Answer from the drawing. Dimensions are ordinates in mm from the lowest x, y and z of the part. Coordinates: 2 decimals unless noted, no trailing zeros. Order: outer loops, then holes, each group sorted by start corner. A loop starts at its lowest first (then second) coordinate and runs counter-clockwise, first axis right, second up. Notation, with made-up numbers: (76, -36) -> (103, -36) arc R16 cw to (103, -14) -> close; hole circle Ø5 at (18.25, 2). An arc over 180 degrees is marked (long way). Answer in a Markdown table with one row per item.
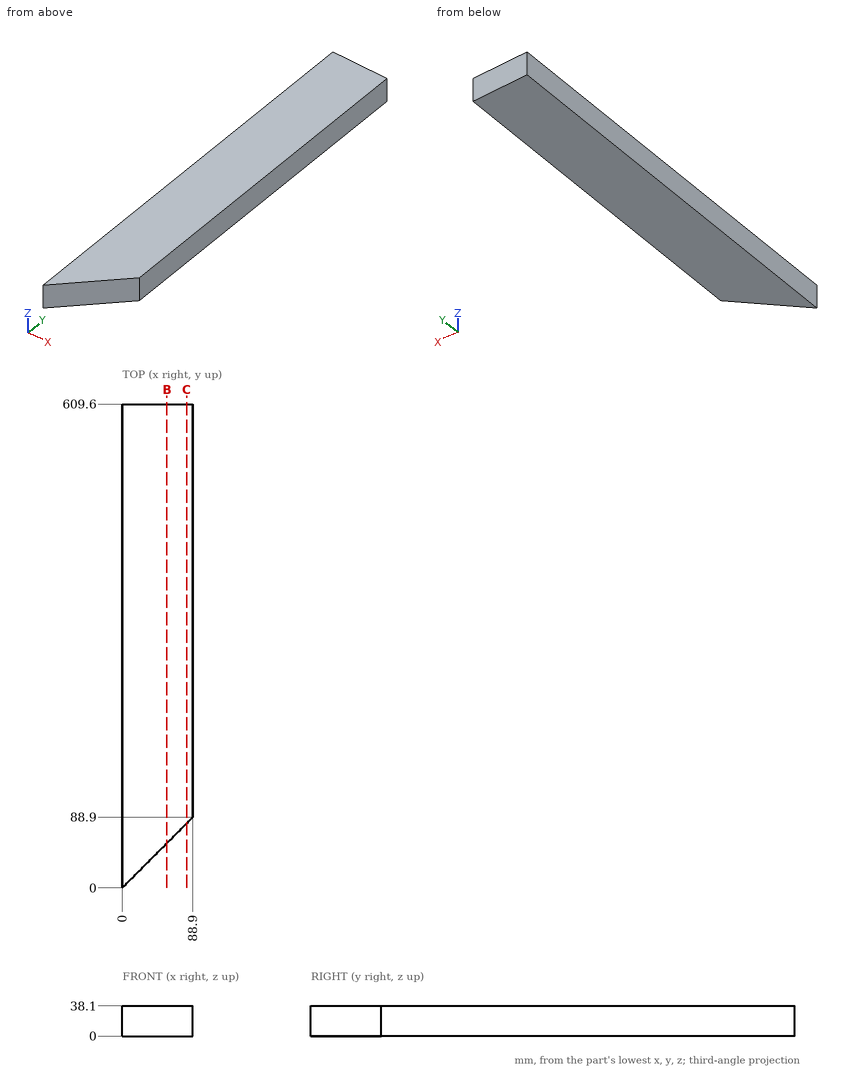
(1) Flat-ended cylindrical pins translate along their axes: pin 1 (8 mm diameter, centred on y = 547.5, z = 18, fed in from -X); pin 2 (3 mm diameter, centred on y = 70, z = 25.5, fed in from +X); pin 3 (4 mm diameter, centred on x = 28.5, z = 4.5, fed in from -Y). Find the tip coordinate at first contact, or state that the pin passes through.
Check values:
| item | result |
|---|---|
| pin 1 | x = 0 |
| pin 2 | x = 71.5 |
| pin 3 | y = 26.5 |
(2) Find the intervals of material crossed by line 1 along Y through (x, z) = (62.5, 18.5); line 2 along Y through (x, z) = (26.5, 8); line 3 along X through (y, z) = (51, 27), in increasing order. Write a range as from..to.
Check values:
| item | result |
|---|---|
| line 1 | 62.5..609.6 |
| line 2 | 26.5..609.6 |
| line 3 | 0..51 |
(3) A cutting plane is placed at B-B, the plane x = 56. Determine the outline of the cut face in (y, z).
Check values:
| item | result |
|---|---|
| outline | (56, 0) -> (609.6, 0) -> (609.6, 38.1) -> (56, 38.1) -> close |
(4) A cutting plane is placed at C-C, the plane x = 81. Determine the outline of the cut face in (y, z), then the cut area to 3 significant figures.
Check values:
| item | result |
|---|---|
| outline | (81, 0) -> (609.6, 0) -> (609.6, 38.1) -> (81, 38.1) -> close |
| area | 20,100 mm² |
